Autodesk Inventor part; units mm, degrees
ref_plane "YZ Plane" through (0, 0, 0) normal (1, 0, 0) x (0, 1, 0)
ref_plane "XZ Plane" through (0, 0, 0) normal (0, 1, 0) x (-1, 0, 0)
ref_plane "XY Plane" through (0, 0, 0) normal (0, 0, 1) x (1, 0, 0)
sketch "Sketch1" plane through (0, 0, 0) normal (0, 1, 0) x (-1, 0, 0)
  circle A0 centre (0, 0) radius 7.62
  line L0 (12.7, 7.62) -> (-12.7, 7.62)
  line L1 (-12.7, 7.62) -> (-12.7, -7.62)
  line L2 (-12.7, -7.62) -> (12.7, -7.62)
  line L3 (12.7, -7.62) -> (12.7, 7.62)
  line L4 (12.7, 7.62) -> (-12.7, -7.62) construction
  line L5 (-12.7, 7.62) -> (12.7, -7.62) construction
  line L6 (12.7, 7.62) -> (38.1, 7.62) construction
  dimension "d0" = 15.24
  dimension "d27" = 25.4
  dimension "d28" = 180
  dimension "d29" = 15.24
extrude "Extrusion1" add sketch "Sketch1" along normal mid plane 25.4
sketch "Sketch2" plane through (0, 12.7, 0) normal (0, 1, 0) x (1, 0, 0)
  circle A0 centre (0, 0) radius 3.175
  dimension "d3" = 6.35
hole "Hole1" at (0, 12.7, 0) direction (0, -1, 0) diameter 10.4648 depth 24.7904 tip angle 118
sketch "Sketch3" plane through (0, 12.7, 0) normal (0, 1, 0) x (1, 0, 0)
  circle A0 centre (0, 0) radius 6.3627
  dimension "d6" = 12.7254
extrude "Extrusion3" cut sketch "Sketch3" against normal blind 11.684
sketch "Sketch4" plane through (0, -12.7, 0) normal (0, -1, 0) x (1, 0, 0)
  circle A0 centre (0, 0) radius 6.3627
  dimension "d9" = 12.7254
extrude "Extrusion4" cut sketch "Sketch4" against normal blind 11.684
sketch "Sketch5" plane through (0, 12.7, 0) normal (0, 1, 0) x (1, 0, 0)
  circle A0 centre (0, 0) radius 6.477
  dimension "d13" = 12.954
extrude "Extrusion5" cut sketch "Sketch5" against normal blind 2.54
sketch "Sketch6" plane through (0, -12.7, 0) normal (0, -1, 0) x (1, 0, 0)
  circle A0 centre (0, 0) radius 6.477
  dimension "d16" = 12.954
extrude "Extrusion6" cut sketch "Sketch6" against normal blind 2.54
sketch "Sketch7" plane through (-12.7, 12.7, 7.62) normal (0, 0, 1) x (1, 0, 0)
  line L0 (3.175, -2.54) -> (22.225, -2.54) construction
  line L1 (22.225, -2.54) -> (22.225, -22.86) construction
  line L2 (22.225, -22.86) -> (3.175, -22.86) construction
  line L3 (3.175, -22.86) -> (3.175, -2.54) construction
  line L4 (3.175, -2.54) -> (22.225, -22.86) construction
  line L5 (22.225, -2.54) -> (3.175, -22.86) construction
  point P0 (12.7, -12.7)
  dimension "d30" = 19.05
  dimension "d31" = 20.32
hole "Hole2" at (9.525, 10.16, 7.62) at (9.525, -10.16, 7.62) at (-9.525, -10.16, 7.62) at (-9.525, 10.16, 7.62) direction (0, 0, -1) diameter 3.2766 end through all
properties part number "brassbushing2" material "Copper"
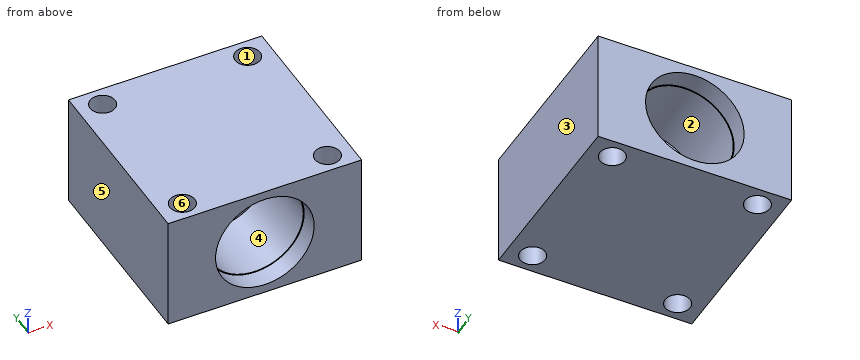
Input: part model. Units: mm. Frame: model coordinates. Face numbers are marked on the shaded views. A direction names the side the tool comes from. Give positions to 0.01 mm unless a question says otherwise; leave off trailing zeros. Order: outer loops, then holes, each group sorted by start corner. A loop starts at its lowest first (then second) coordinate and runs counter-clockwise, first axis right, second up.
1. Cut plane B-B (x = 0). Return loops of the section in (y, z).
Computed:
outline: (-12.7, -7.62) - (12.7, -7.62) - (12.7, -6.48) - (10.16, -6.48) - (10.16, -6.36) - (1.02, -6.36) - (1.02, -5.23) - (-1.02, -5.23) - (-1.02, -6.36) - (-10.16, -6.36) - (-10.16, -6.48) - (-12.7, -6.48) - close; (-12.7, 6.48) - (-10.16, 6.48) - (-10.16, 6.36) - (-1.02, 6.36) - (-1.02, 5.23) - (1.02, 5.23) - (1.02, 6.36) - (10.16, 6.36) - (10.16, 6.48) - (12.7, 6.48) - (12.7, 7.62) - (-12.7, 7.62) - close
2. Line query: probe 1 along X at (y, z) = (10.25, 2.75); probe 2 along X at (y, z) = (6.25, 0); probe 3 along Z at (x, y) = (0, 12). Output: solid intervals per line, ascending.
Computed:
probe 1: x = -12.7 to -11.16, -7.89 to -5.86, 5.86 to 7.89, 11.16 to 12.7
probe 2: x = -12.7 to -6.36, 6.36 to 12.7
probe 3: z = -7.62 to -6.48, 6.48 to 7.62
3. Cut plane C-C (y = -4). Return loops of the section in (x, z).
Computed:
outline: (-12.7, -7.62) - (12.7, -7.62) - (12.7, 7.62) - (-12.7, 7.62) - close; hole circle Ø12.73 at (0, 0)
4. Draft query along X for the marked faces 3, 4, 5 and 6. Return one class per face: released by +X, released by -X, zero draft, split by the parting line, or undercut.
Computed:
face 3: released by +X
face 4: undercut
face 5: released by -X
face 6: undercut
5. Cut plane D-D (z = -5.75). Return loops of the section in (x, y) (3 decimals), and give its area (3 significant figures).
Computed:
outline: (-12.7, -12.7) - (-2.981, -12.7) - (-2.981, -10.16) - (-2.724, -10.16) - (-2.724, -1.016) - (2.724, -1.016) - (2.724, -10.16) - (2.981, -10.16) - (2.981, -12.7) - (12.7, -12.7) - (12.7, 12.7) - (2.981, 12.7) - (2.981, 10.16) - (2.724, 10.16) - (2.724, 1.016) - (-2.724, 1.016) - (-2.724, 10.16) - (-2.981, 10.16) - (-2.981, 12.7) - (-12.7, 12.7) - close; hole circle Ø3.277 at (-9.525, -10.16); hole circle Ø3.277 at (-9.525, 10.16); hole circle Ø3.277 at (9.525, -10.16); hole circle Ø3.277 at (9.525, 10.16)
area: 481 mm2
6. Cut plane A-A (z = 0.75). Return loops of the section in (x, y) (3 decimals), and give its area (3 significant figures).
Computed:
outline: (-12.7, -12.7) - (-6.433, -12.7) - (-6.433, -10.16) - (-6.318, -10.16) - (-6.318, -1.016) - (-5.178, -1.016) - (-5.178, 1.016) - (-6.318, 1.016) - (-6.318, 10.16) - (-6.433, 10.16) - (-6.433, 12.7) - (-12.7, 12.7) - close; (5.178, -1.016) - (6.318, -1.016) - (6.318, -10.16) - (6.433, -10.16) - (6.433, -12.7) - (12.7, -12.7) - (12.7, 12.7) - (6.433, 12.7) - (6.433, 10.16) - (6.318, 10.16) - (6.318, 1.016) - (5.178, 1.016) - close; hole circle Ø3.277 at (-9.525, -10.16); hole circle Ø3.277 at (-9.525, 10.16); hole circle Ø3.277 at (9.525, -10.16); hole circle Ø3.277 at (9.525, 10.16)
area: 294 mm2
7. Pin query (flat end, axial travel): pin 1 Ø4 at (x, z) = (1.5, 0) entering from -Y. Return the tip coordinate at first contact, or that it passes through.
Computed:
pin 1: passes through
8. Set-up query: the marked faces 1 and 2. Return all of +Z, -Z, +X, -X, +Y, -Y with unobstructed straight access to the full face (end or side cutting, diameter ignored); none if empty.
Computed:
face 1: +Z, -Z
face 2: +Y
